Autodesk Inventor part; units mm, degrees
ref_plane "YZ Plane" through (0, 0, 0) normal (1, 0, 0) x (0, 1, 0)
ref_plane "XZ Plane" through (0, 0, 0) normal (0, 1, 0) x (-1, 0, 0)
ref_plane "XY Plane" through (0, 0, 0) normal (0, 0, 1) x (1, 0, 0)
sketch "Esquisse1" plane through (0, 0, 0) normal (0, 0, 1) x (1, 0, 0)
  circle A0 centre (0, 0) radius 9.9
  circle A1 centre (0, 0) radius 5
  dimension "d0" = 19.8
  dimension "d1" = 10
extrude "Extrusion1" add sketch "Esquisse1" along normal blind 50
sketch "Esquisse2" plane through (0, 0, 0) normal (0, 1, 0) x (-1, 0, 0)
  line L0 (0, 0) -> (0, 5)
  line L1 (9.9, 50) -> (-9.9, 50)
  line L2 (0, 50) -> (0, 45)
  dimension "d4" = 5
  dimension "d5" = 5
hole "Perçage1" at (0, 0, 5) at (0, 0, 45) direction (0, -1, 0) diameter 4 end through all both
sketch "Esquisse3" plane through (0, 0, 50) normal (0, 0, 1) x (1, 0, 0)
  circle A0 centre (0, 0) radius 9.9
  circle A1 centre (0, 0) radius 5
sketch "Esquisse4" plane through (0, 0, 50) normal (0, 0, 1) x (1, 0, 0)
  point P0 (0, 0)
extrude "Extrusion2" add sketch "Esquisse3" along normal blind 5
properties part number "tube vers bogie"
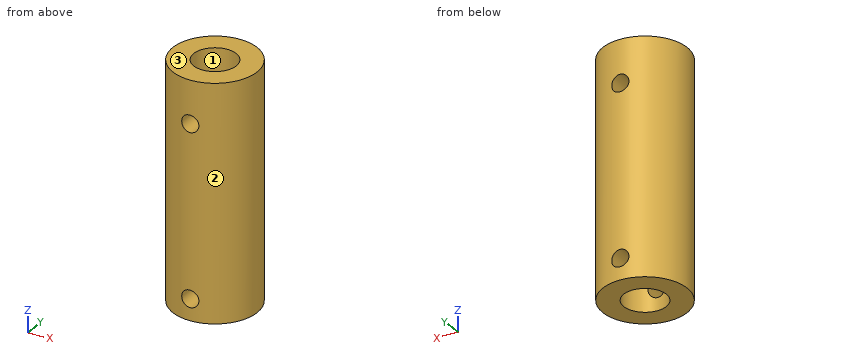
For this review, take the finished solid that the model builds, in its own axes (mm). Face numbers are marked on the shaded views. Give positions to 0.01 mm unless a question says otherwise; leave off trailing zeros. Loops run counter-clockwise (first coordinate to the right, second up) from the corner with the lowest first, then second, coordinate; pieces in that order, holes last.
Item 1: Take a section at A-A, the plane y = 0. State the section outline as (x, z) points.
Item 2: Take a section at B-B, the plane x = 0. State the section outline as (y, z) points.
Item 3: Take a section at D-D, the plane y = -8.25. State the section outline as (x, z) points, and give its area (3 significant figures).
Item 4: Take a section at C-C, the plane z = 45. State the section outline as (x, y) points.
Item 5: For line 1 along Z through (x, y) = (0, -8.6); line 2 along Y through (x, z) = (0, 14); line 3 along X through (y, z) = (4, 3), list the stretches that pass through material, from the lowest coordinate up.
Item 6: Insertion check: pin 1 (3 mm diameter, centred on x = 0, z = 5, fed in from +Y); pin 2 (2 mm diameter, centred on y = 8, z = 35, fed in from +X); pin 3 (2 mm diameter, centred on x = 7, z = 15.5, fed in from -Y); pin 4 (3 mm diameter, centred on x = -3, z = 43, fed in from -Y). Each pin has a flat end and moves straight along its axis. Give the tip position at first contact, or say it passes through.
Item 7: Draft analysis for pull direction Y (two halves, no side actions). For the marked faces 1, 2 and 3, state which applies: +Y half, -Y half, draft (parallel to the pull), parting line (faces both ways), or undercut.
Calculated:
1. outline: (-9.9, 0) - (-5, 0) - (-5, 55) - (-9.9, 55) - close; (5, 0) - (9.9, 0) - (9.9, 55) - (5, 55) - close
2. outline: (-9.9, 0) - (-5, 0) - (-5, 3) - (-9.9, 3) - close; (-9.9, 7) - (-5, 7) - (-5, 43) - (-9.9, 43) - close; (-9.9, 47) - (-5, 47) - (-5, 55) - (-9.9, 55) - close; (5, 0) - (9.9, 0) - (9.9, 3) - (5, 3) - close; (5, 7) - (9.9, 7) - (9.9, 43) - (5, 43) - close; (5, 47) - (9.9, 47) - (9.9, 55) - (5, 55) - close
3. outline: (-5.47, 0) - (5.47, 0) - (5.47, 55) - (-5.47, 55) - close; hole circle Ø4 at (0, 5); hole circle Ø4 at (0, 45)
3. area: 577 mm2
4. outline: (-2, -9.7) - (-2, -4.58) arc R5 cw to (-2, 4.58) - (-2, 9.7) arc R9.9 ccw to start; (2, -9.7) arc R9.9 ccw to (2, 9.7) - (2, 4.58) arc R5 cw to (2, -4.58) - close
5. line 1: z = 0 to 3, 7 to 43, 47 to 55
5. line 2: y = -9.9 to -5, 5 to 9.9
5. line 3: x = -9.06 to -3, 3 to 9.06
6. pin 1: passes through
6. pin 2: stops at x = 7
6. pin 3: stops at y = -7.87
6. pin 4: stops at y = -9.79
7. face 1: undercut
7. face 2: parting line
7. face 3: draft
